Build history of the part. All positions in model axes, mm. A direction names the side the tool comes from. Round coordinates to 2 decimals unless told otherwise and drop trailing zeros. Loops run counter-clockwise (first coordinate to the right, second up) from the corner with the lowest first, then second, coordinate; pieces in that order, holes last. Notation, with made-up numbers: M 74,85 L 83,85 A31 cw 83,115 Z; hole C 62.25,62 d2. An arc over 180 degrees is marked long. Use one line per item in the form item = value. Start each with the question number.
```python
from build123d import *

# Parameters (mm, degrees)
F0_R     = 1.75
F1_DEPTH = 30
F2_DEPTH = 2
F3_START = 28
F3_DEPTH = 2


# Not quite as in the source:
# - ends of sketch curves that miss each other by under 0.0002 mm in the source are joined


with BuildPart() as f1:
    # F0 (on Top) → F1 (new body)
    with BuildSketch(Plane.XY):
        Polygon((-10, -17.3205080757), (10, -17.3205080757), (13.500000035, -11.2583301886), (9.5000001398, -11.2583302492), (14.5000001398, -2.5980762114), (16.5000001398, -6.0621778265), (20, 0), (10, 17.3205080757), (3, 17.3205080757), (5, 13.8564064606), (-5, 13.8564064606), (-3, 17.3205080757), (-10, 17.3205080757), (-20, 0), (-16.4999999301, -6.0621779476), (-14.4999999301, -2.5980763325), (-9.4999999301, -11.2583303703), (-13.4999999301, -11.2583303703), align=None)
        Circle(F0_R, mode=Mode.SUBTRACT)
    extrude(amount=F1_DEPTH)

    # F0 (on Top) → F2 (join)
    with BuildSketch(Plane.XY):
        Polygon((-16.4999999301, -6.0621779476), (-13.4999999301, -11.2583303703), (-9.4999999301, -11.2583303703), (-14.4999999301, -2.5980763325), align=None)
        Polygon((5, 13.8564064606), (3, 17.3205080757), (-3, 17.3205080757), (-5, 13.8564064606), align=None)
        Polygon((9.5000001398, -11.2583302492), (13.5000001398, -11.2583302492), (16.500000035, -6.0621777659), (14.5000001398, -2.5980762114), align=None)
    extrude(amount=F2_DEPTH)

    # F0 (on Top) → F3 (join)
    with BuildSketch(Plane.XY.offset(F3_START)):
        Circle(F0_R)
    extrude(amount=F3_DEPTH)


solid = f1.part
```
Q1. Saw through at D-D (y = -5.5). Give the cut face in (x, z).
Q2. Saw through at C-C (y = -10). Give the cut face in (x, z), and give its area (3 significant figures).
Q3. Saw through at B-B (x = 0). Give the cut face in (y, z), and give its area (3 significant figures).
Q4. Drop flat-ended pins along their axis: P1, Ø10, axis at y = -3.5, z = 20, coming from the -X side; P2, Ø1.7, axis at x = -1, y = 16.5, coming from the +Z side; P3, Ø1.8, axis at x = 0.5, y = -0.5, coming from the -Z side. Give the stop position or say it passes through.
Q5. Tool access for faces 4 (the face through (12, -11.258, 16)), 5 (the face through (-11, -11.258, 16)), 6 (the face through (15.49, -4.31, 15.8)), 7 (the face through (-13, -8, 2)): list every direction of +Z, -Z, +X, -X, +Y, -Y with a clear straight run to the whole face (end or side of a thin tool).
Q6. Pull direction X, two halves, no side cores. Call faces 1 (the face through (4, 0, 0)), 2 (the face through (-4.014, 15.564, 15.804)), 3 (the face through (-14.93, 8.78, 14.79)): pulls with the +X half, pulls with the -X half, needs draft (parallel to the pull), parting line crosses it, or undercut.
Q7. Saw through at A-A (z = 6.5). Give the cut face in (x, y), and give its area (3 significant figures).
Q8. Wall check: probe 1 along Y at (x, z) = (0, 18.75); probe 2 along X at (y, z) = (-5, 16.5); probe 3 along X at (y, z) = (-4, 15.25). Give the ranges that are in metal, low to high.
Filled in:
q1.outline = M -16.82,0 L 16.82,0 L 16.82,30 L 16.18,30 L 16.18,2 L 12.82,2 L 12.82,30 L -12.82,30 L -12.82,2 L -16.18,2 L -16.18,30 L -16.82,30 Z
q2.outline = M -14.23,0 L 14.23,0 L 14.23,2 L 10.23,2 L 10.23,30 L -10.23,30 L -10.23,2 L -14.23,2 Z
q2.area = 630 mm²
q3.outline = M -17.32,0 L -1.75,0 L -1.75,28 L 1.75,28 L 1.75,0 L 17.32,0 L 17.32,2 L 13.86,2 L 13.86,30 L -17.32,30 Z
q3.area = 844 mm²
q4.P1 = -20
q4.P2 = 2
q4.P3 = 28
q5.face_4 = +Z, +X
q5.face_5 = +Z, -X
q5.face_6 = +Z, -Y
q5.face_7 = +Z
q6.face_1 = needs draft
q6.face_2 = undercut
q6.face_3 = pulls with the -X half
q7.outline = M -20,0 L -16.5,-6.06 L -14.5,-2.6 L -9.5,-11.26 L -13.5,-11.26 L -10,-17.32 L 10,-17.32 L 13.5,-11.26 L 9.5,-11.26 L 14.5,-2.6 L 16.5,-6.06 L 20,0 L 10,17.32 L 3,17.32 L 5,13.86 L -5,13.86 L -3,17.32 L -10,17.32 Z; hole C 0,0 d3.5
q7.area = 946 mm²
q8.probe_1 = -17.32 to -1.75, 1.75 to 13.86
q8.probe_2 = -17.11 to -15.89, -13.11 to 13.11, 15.89 to 17.11
q8.probe_3 = -17.69 to -15.31, -13.69 to 13.69, 15.31 to 17.69
